Could you check a few things on this drawing? It's one solid part, dimensions in mm from its lowest x, y, z. A direction names the side the tool comes from. Round coordinates to 2 decimals unless told otherwise and drop trailing zeros. Loops run counter-clockwise (first coordinate to the right, second up) from the corner with the lowest first, then second, coordinate; pieces in that order, holes last. Notation, with made-up numbers: M -3,29.25 L 27,29.25 A12 ccw 27,36.25 Z; hole C 86.25,56.5 d9. An arc over 180 degrees is marked long. Write item = value, one per line. Start each with the question number.
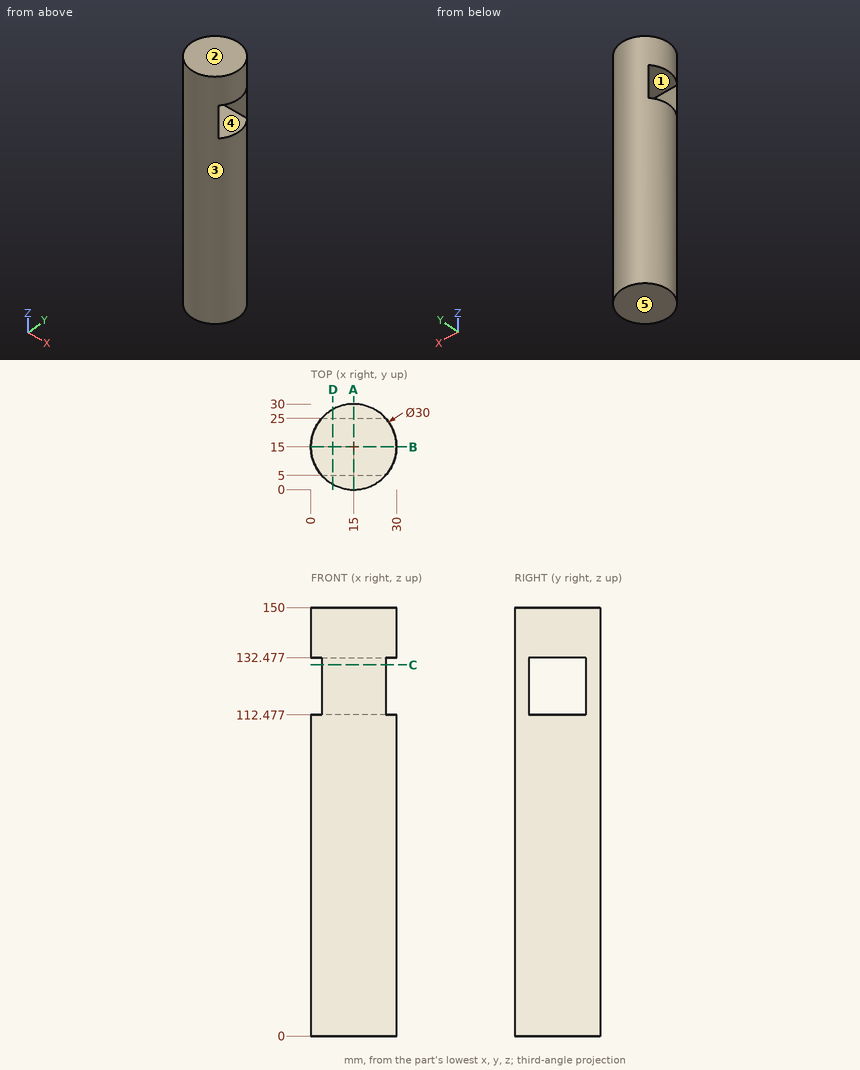
Item 1: Please list where these lines run through material, in increasing order: line 1 (Z direction, x = 1.75, y = 11); line 2 (X direction, y = 15.25, z = 98); line 3 (Y direction, x = 13, z = 124) (1 decimal). Write a range as [from, to].
Item 2: Will these pins go through, and if not, where does the flat tip stop? pin 1 Ø6 at (y, z) = (21, 51) entering from +X; pin 2 Ø10 at (x, z) = (23.5, 50) entering from +Y; pin 3 Ø3 at (x, z) = (3.5, 79) entering from -Y.
Item 3: For the marked faces 1 and 2, which set-ups out of +Z, -Z, +X, -X, +Y, -Y let a thin tool reach every point of the face, with its end or its side?
Item 4: I want a section at C-C, the plane z = 130. List the corners of the cut face in (x, y) for me, then the cut area to 3 significant figures.
Item 5: We'd pull the mould along Y, two halves only. Please class the marked faces 3, 4 and 5: released by +Y, released by -Y, zero draft, split by the parting line, or undercut.
Item 6: I want a section at B-B, the plane y = 15. List the corners of the cut face in (x, z) for me, then the cut area to 3 significant figures.
Item 7: I want a section at D-D, the plane x = 7.75. List the corners of the cut face in (y, z) for me, then the cut area to 3 significant figures.
Item 8: I want a section at A-A, the plane x = 15. List the corners of the cut face in (y, z) for me.
Worked out:
q1.line_1 = [0, 112.48], [132.48, 150]
q1.line_2 = [0, 30]
q1.line_3 = [0.1, 5], [25, 29.9]
q2.pin_1 = 29.7
q2.pin_2 = 29.59
q2.pin_3 = 3.82
q3.face_1 = +X, -X
q3.face_2 = +Z, +X, -X, +Y, -Y
q4.outline = M 3.82,5 A15 ccw 26.18,5 Z; M 3.82,25 L 26.18,25 A15 ccw Z
q4.area = 155 mm2
q5.face_3 = split by the parting line
q5.face_4 = undercut
q5.face_5 = zero draft
q6.outline = M 0,0 L 30,0 L 30,112.48 L 0,112.48 Z; M 0,132.48 L 30,132.48 L 30,150 L 0,150 Z
q6.area = 3,900 mm2
q7.outline = M 1.87,0 L 28.13,0 L 28.13,150 L 1.87,150 Z; hole M 5,112.48 L 25,112.48 L 25,132.48 L 5,132.48 Z
q7.area = 3,540 mm2
q8.outline = M 0,0 L 30,0 L 30,150 L 0,150 Z; hole M 5,112.48 L 25,112.48 L 25,132.48 L 5,132.48 Z
